Geometry: final body of the model. Coordinates: model frame, mm. Round coordinates to 2 decimals unless told otherwise and drop trailing zeros. Loops run counter-clockwise (first coordinate to the right, second up) from the corner with the lowest first, then second, coordinate; pieces in that order, holes last. Notation, with made-up numbers: (53, 43.25) - (82, 43.25) arc R12 ccw to (82, 65.25) - close; hole circle Ø2 at (68.25, 67). An arc over 180 degrees is marked (long way). Return JSON: item names as keys, results as strings. Group by question number.
1. First-contact query: pin 1 Ø3 at (x, z) = (-209.5, 31.5) entering from -Y; pin 2 Ø8 at (x, z) = (87, 22) entering from +Y; pin 3 Ø5 at (x, z) = (-79, 18.5) entering from -Y; pin 4 Ø12 at (x, y) = (100, 719.5) entering from -Z. Flat tips, straight axial feed; report the tip coordinate or a pass-through.
2. Section B-B on y = 138. Return loops of the section in (x, z), and give its area (3 significant figures).
3. Section C-C on x = 247.5. Return loops of the section in (y, z).
4. Section A-A on z = 8. Return loops of the section in (x, y).
5. Material intervals for probe 1 along Y at (x, z) = (37.5, 9.5); probe 2 along Y at (x, z) = (49, 4); probe 3 along X at (y, z) = (263.5, 30), sorted ascending.
Autodesk Inventor part; units mm, degrees
ref_plane "YZ Plane" through (0, 0, 0) normal (1, 0, 0) x (0, 1, 0)
ref_plane "XZ Plane" through (0, 0, 0) normal (0, 1, 0) x (-1, 0, 0)
ref_plane "XY Plane" through (0, 0, 0) normal (0, 0, 1) x (1, 0, 0)
sketch "Sketch1" plane through (0, 0, 0) normal (0, 0, 1) x (1, 0, 0)
  line L0 (-571.5, -1549.4) -> (571.5, -1549.4)
  line L1 (571.5, -1549.4) -> (571.5, 1549.4)
  line L2 (571.5, 1549.4) -> (-571.5, 1549.4)
  line L3 (-571.5, 1549.4) -> (-571.5, -1549.4)
  line L4 (-571.5, -1549.4) -> (571.5, 1549.4) construction
  line L5 (571.5, -1549.4) -> (-571.5, 1549.4) construction
  line L6 (-571.5, 0) -> (571.5, 0)
  line L7 (571.5, 0) -> (-571.5, -1549.4)
  line L8 (-535.73, -1575.7877) -> (-607.27, -1523.0123)
  line L9 (607.27, -26.3877) -> (535.73, 26.3877)
  line L10 (535.73, 26.3877) -> (-607.27, -1523.0123)
  line L11 (-535.73, -1575.7877) -> (607.27, -26.3877)
  line L12 (535.73, 26.3877) -> (571.5, 74.8759)
  line L13 (-571.5, 1549.4) -> (571.5, -1549.4) construction
  line L14 (571.5, 0) -> (-571.5, 1549.4)
  line L15 (-535.73, 1575.7877) -> (-607.27, 1523.0123)
  line L16 (607.27, 26.3877) -> (535.73, -26.3877)
  line L17 (535.73, -26.3877) -> (-607.27, 1523.0123)
  line L18 (-535.73, 1575.7877) -> (607.27, 26.3877)
  line L19 (535.73, -26.3877) -> (571.5, -74.8759)
  point P0 (0, 0)
  point P1 (571.5, 74.8759)
  point P2 (-516.2637, 1549.4)
  point P3 (-571.5, 1474.5241)
  point P4 (571.5, -74.8759)
  point P5 (571.5, -74.8759)
  point P6 (516.2637, 0)
  point P7 (-571.5, -1474.5241)
  point P8 (-516.2637, -1549.4)
  point P9 (543.8818, -37.438)
  point P10 (571.5, 0)
  point P11 (571.5, 0)
  point P12 (516.2637, 0)
  point P13 (571.5, 0)
  point P14 (-571.5, 1549.4)
  point P15 (543.8818, 37.438)
  point P16 (571.5, 74.8759)
  point P17 (571.5, -74.8759)
  point P18 (571.5, 0)
  point P19 (-571.5, -1549.4)
  point P20 (516.2637, 0)
  point P21 (571.5, 0)
  point P22 (-571.5, 1549.4)
  point P23 (571.5, 0)
  point P24 (-571.5, -1549.4)
  dimension "d0" = 1143
  dimension "d1" = 3098.8
  dimension "d3" = 88.9
  dimension "d4" = 88.9
extrude "Extrusion1" add sketch "Sketch1" along normal blind 38.1 contours L19 L16 L7 | L7 L1 L19 | L10 L9 L6 | L17 L3 L14 L12 L10 | L6 L16 L17 | L14 L12 L1 | L9 L12 L14 | L12 L14 L2 L18
properties part number "S_2x4x78.175"
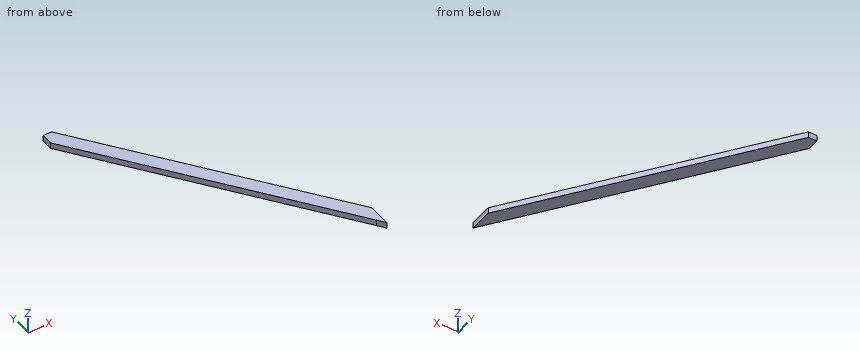
Taken from the geometry:
{
 "1": {"pin 1": "y = 981.78", "pin 2": "y = 737.06", "pin 3": "y = 803.52", "pin 4": "z = 0"},
 "2": {"outline": "(414.46, 0) - (524.93, 0) - (524.93, 38.1) - (414.46, 38.1) - close", "area": "4,210 mm2"},
 "3": {"outline": "(364.32, 0) - (514.08, 0) - (514.08, 38.1) - (364.32, 38.1) - close"},
 "4": {"outline": "(-571.5, 1474.52) - (535.73, -26.39) - (571.5, -74.88) - (571.5, 74.88) - (-516.26, 1549.4) - (-571.5, 1549.4) - close"},
 "5": {"probe 1": "648.99 to 798.74", "probe 2": "633.4 to 783.15", "probe 3": "321.88 to 432.35"}
}
